The listing builds one solid part. Answer for the finished solid, in the listing's coordinates (mm). A direction names the side the tool comes from. Coordinates: 2 decimals unless noted, no trailing zeros. Write each loop counter-clockwise with the first axis right and the second up, starting at its lowest first coordinate (ties: lowest second). Pieces come first, ordered by that corner, then holes.
```python
from build123d import *

# Parameters (mm, degrees)
F2_DEPTH = 99.06
F4_D     = 9.92124
F4_DEPTH = 41.91
F4_TIP   = 2.980641204


with BuildPart() as f1:
    # F0 (on Front) → F1 (revolve)
    with BuildSketch(Plane.XZ):
        Polygon((0, 11.43), (0, 0), (11.43, 0), align=None)
    revolve(axis=Axis((0, 0, 5.715), (0, 0, 1)))

    # F2 (add): a face of the model
    f2_faces = [f1.faces().sort_by_distance(p)[0] for p in [
        (0, 0, 0),
    ]]
    extrude(f2_faces, amount=F2_DEPTH)

    # F4
    with Locations(Plane(origin=(0, 0, -99.06), x_dir=(1, 0, 0), z_dir=(0, 0, -1))):
        with Locations((0, 0)):
            Hole(F4_D / 2, depth=F4_DEPTH)
            with Locations((0, 0, -(F4_DEPTH + F4_TIP / 2))):  # 118° drill point
                Cone(0, F4_D / 2, F4_TIP, mode=Mode.SUBTRACT)


solid = f1.part
```
(1) Each of these flat-tipped pins is pushed along its axis until it touches: pin 1 (6 mm diameter, centred on x = 0.5, z = -30.5, fed in from +Y); pin 2 (3 mm diameter, centred on x = -3.5, y = 7.5, fed in from +Z); pin 3 (1.5 mm diameter, centred on y = -8.5, z = -68, fed in from -X); pin 4 (1.5 mm diameter, centred on x = 0.5, y = 3, fed in from -Z). Where does it stop, or does it pass through?
(2) Which of the six approach directions +Z, -Z, +X, -X, +Y, -Y give full straight-line access (tool end or side, diameter ignored) to faces 1 (the cylindrical face through (1.08, 4.84, -77.81)), 2 (the conical face through (-2.456, -1.883, 8.335))?
(3) Find the intervals of material crossed by probe 1 along X at (y, z) = (-1, -59); probe 2 along Y at (x, z) = (-2, -72); probe 3 along Z at (x, y) = (-7, -7.5), in increasing order.
(4) For a pull along Y with two mould halves and no side action, classify faces 3 (the cylindrical face through (10.902, 3.433, -48.837)), 4 (the conical face through (-0.187, 0.841, -54.687)), 5 (the flat face through (-2, -5, -99.06)) as pulls with the +Y half, pulls with the -Y half, needs draft (parallel to the pull), parting line crosses it, or undercut.
(5) Section A-A, the plane z = -17.5 is taken. Write down the section's boundary in (x, y), plus the area to 3 significant figures.
(6) Section B-B, the plane z = -87.5 is taken. Write down the section's boundary in (x, y).
Solution:
1. pin 1: stops at y = 11.43
1. pin 2: stops at z = 4.65
1. pin 3: stops at x = -8.4
1. pin 4: stops at z = -56.45
2. face 1: -Z
2. face 2: +Z
3. probe 1: x = -11.39 to -4.86, 4.86 to 11.39
3. probe 2: y = -11.25 to -4.54, 4.54 to 11.25
3. probe 3: z = -99.06 to 1.17
4. face 3: parting line crosses it
4. face 4: undercut
4. face 5: needs draft
5. outline: circle Ø22.86 at (0, 0)
5. area: 410 mm2
6. outline: circle Ø22.86 at (0, 0); hole circle Ø9.92 at (0, 0)
